Could you check a few things on this model? Use its own coordinates, in mm. A direction names the side the tool comes from. Coordinates: 2 decimals unless noted, no trailing zeros. Write each loop counter-clockwise with the first axis right and the second up, starting at its lowest first coordinate (ties: lowest second). Pieces come first, ordered by that corner, then holes.
Item 1: For P1, Ø5, axis at x = 0, z = 34, coming from the +Y side; P2, Ø2, axis at y = 0, z = -80, coming from the +X side; P3, Ø3, axis at x = 0, y = 0, coming from the +Z side; P4, Ø3, axis at x = 0, y = 0, coming from the -Z side, each with a flat end and sliding along its axis, tell me the tip position at first contact or that it passes through.
Item 2: Thinking about a two-plate mould opening in Y: for faces 1 (the flat face through (0, -5, -72)), 2 (the flat face through (2, 0.1, -32)), 3 (the cylindrical face through (-0.07, 0.07, -81.65)), 4 (the conical face through (0.3, 0.1, 93.7)), which applies, +Y half, -Y half, draft (parallel to the pull), parting line (faces both ways), or undercut?
Item 3: Which directions (+Z, -Z, +X, -X, +Y, -Y) give clear straight access to the entire face, cutting with the end or side of a thin tool? Please do faces 5 (the cylindrical face through (-1.216, 1.115, -100.17)), 6 (the flat face through (2, 0.1, 36)), 7 (the cylindrical face through (1.216, 1.115, 100.17)), 8 (the flat face through (2.3, -2, -33.9)), 9 (the flat face through (2, 0, -106)).
Item 4: I want a section at B-B on z = -34. Please give me the cut outline in (x, y).
Item 5: If I drill on probe 1 along Z at (x, y) = (0, 3.8); probe 2 along Z at (x, y) = (2.5, -4); probe 3 along X at (y, z) = (-1.4, 34), over which ranges is the centre line in solid material (lowest first)?
Item 6: I want a section at A-A on z = -4. Please give me the cut outline in (x, y), then the cut area to 3 significant figures.
from build123d import *

# Parameters (mm, degrees)
ESQUISSE1_W                                        = 10
ESQUISSE1_H                                        = 10
BOSS_EXTRU_1_DEPTH                                 = 106
TROU_TARAUD_M41_D                                  = 3.3
TROU_TARAUD_M41_DEPTH                              = 11.5
TROU_TARAUD_M41_TIP                                = 0.991420021
TROU_TARAUD_M42_D                                  = 3.3
TROU_TARAUD_M42_DEPTH                              = 11.5
TROU_TARAUD_M42_TIP                                = 0.991420021
CONG_1_R                                           = 2
CHAMBRAGE_POUR_VIS_T_TE_HEXAGONALE_M41_D           = 4.3
CHAMBRAGE_POUR_VIS_T_TE_HEXAGONALE_M41_CBORE_D     = 8
CHAMBRAGE_POUR_VIS_T_TE_HEXAGONALE_M41_CBORE_DEPTH = 4.9
ENL_V_MAT_EXTRU_1_REACH                            = 108.588
ESQUISSE8_W                                        = 10
ESQUISSE8_H                                        = 8
TROU_TARAUD_M44_D                                  = 3.3


with BuildPart() as part:
    # Esquisse1 → Boss.-Extru.1 (new, symmetric)
    with BuildSketch(Plane.XY):
        Rectangle(ESQUISSE1_W, ESQUISSE1_H)
    extrude(amount=BOSS_EXTRU_1_DEPTH, both=True)

    # Trou taraudé M41
    with Locations(Plane.XY.offset(106)):
        with Locations((0, 0)):
            Hole(TROU_TARAUD_M41_D / 2, depth=TROU_TARAUD_M41_DEPTH)
            with Locations((0, 0, -(TROU_TARAUD_M41_DEPTH + TROU_TARAUD_M41_TIP / 2))):  # 118° drill point
                Cone(0, TROU_TARAUD_M41_D / 2, TROU_TARAUD_M41_TIP, mode=Mode.SUBTRACT)

    # Trou taraudé M42
    with Locations(Plane(origin=(0, 0, -106), x_dir=(-1, 0, 0), z_dir=(0, 0, -1))):
        with Locations((0, 0)):
            Hole(TROU_TARAUD_M42_D / 2, depth=TROU_TARAUD_M42_DEPTH)
            with Locations((0, 0, -(TROU_TARAUD_M42_DEPTH + TROU_TARAUD_M42_TIP / 2))):  # 118° drill point
                Cone(0, TROU_TARAUD_M42_D / 2, TROU_TARAUD_M42_TIP, mode=Mode.SUBTRACT)

    # Congé1
    cong_1_edges = [part.edges().sort_by_distance(p)[0] for p in [
        (-5, 5, 0),
        (5, 5, 0),
        (5, -5, 0),
        (-5, -5, 0),
    ]]
    fillet(cong_1_edges, radius=CONG_1_R)

    # Chambrage pour vis à tête hexagonale M41 (through all)
    with Locations(Plane(origin=(0, 5, 0), x_dir=(1, 0, 0), z_dir=(0, 1, 0))):
        with Locations((0, 34), (0, -34)):
            CounterBoreHole(CHAMBRAGE_POUR_VIS_T_TE_HEXAGONALE_M41_D / 2, CHAMBRAGE_POUR_VIS_T_TE_HEXAGONALE_M41_CBORE_D / 2, CHAMBRAGE_POUR_VIS_T_TE_HEXAGONALE_M41_CBORE_DEPTH)

    # Esquisse8 → Enlèv. mat.-Extru.1 (cut, up to next)
    with BuildSketch(Plane(origin=(5, 0, 0), x_dir=(0, 0, -1), z_dir=(1, 0, 0)), mode=Mode.PRIVATE) as enl_v_mat_extru_1_sk1:
        with Locations((34, -6)):
            Rectangle(ESQUISSE8_W, ESQUISSE8_H)
    enl_v_mat_extru_1_tool1 = extrude(enl_v_mat_extru_1_sk1.sketch, amount=-ENL_V_MAT_EXTRU_1_REACH, mode=Mode.PRIVATE) & part.part
    # Esquisse8 → Enlèv. mat.-Extru.1 (cut, up to next)
    with BuildSketch(Plane(origin=(5, 0, 0), x_dir=(0, 0, -1), z_dir=(1, 0, 0)), mode=Mode.PRIVATE) as enl_v_mat_extru_1_sk2:
        with Locations((-34, -6)):
            Rectangle(ESQUISSE8_W, ESQUISSE8_H)
    enl_v_mat_extru_1_tool2 = extrude(enl_v_mat_extru_1_sk2.sketch, amount=-ENL_V_MAT_EXTRU_1_REACH, mode=Mode.PRIVATE) & part.part
    add(enl_v_mat_extru_1_tool1.solids().sort_by_distance((5, -6, -34))[0], mode=Mode.SUBTRACT)
    add(enl_v_mat_extru_1_tool2.solids().sort_by_distance((5, -6, 34))[0], mode=Mode.SUBTRACT)

    # Trou taraudé M44 (through all)
    with Locations(Plane(origin=(5, 0, 0), x_dir=(0, 0, -1), z_dir=(1, 0, 0))):
        with Locations((-80, 0), (80, 0)):
            Hole(TROU_TARAUD_M44_D / 2)


solid = part.part
Response values:
1. P1: stops at y = 0.1
1. P2: passes through
1. P3: stops at z = 94.41
1. P4: stops at z = -94.41
2. face 1: -Y half
2. face 2: +Y half
2. face 3: undercut
2. face 4: undercut
3. face 5: -Z
3. face 6: +Y
3. face 7: +Z
3. face 8: +X, -X, -Y
3. face 9: -Z, +X, -X, +Y, -Y
4. outline: (-5, -2) - (-2.15, -2) - (-2.15, 0.1) - (-4, 0.1) - (-4, 4.73) arc R2 ccw to (-5, 3) - close; (2.15, -2) - (5, -2) - (5, 3) arc R2 ccw to (4, 4.73) - (4, 0.1) - (2.15, 0.1) - close
5. probe 1: z = -106 to -38, -30 to 30, 38 to 106
5. probe 2: z = -106 to -39, -29 to 29, 39 to 106
5. probe 3: x = -5 to -2.15, 2.15 to 5
6. outline: (-5, -3) arc R2 ccw to (-3, -5) - (3, -5) arc R2 ccw to (5, -3) - (5, 3) arc R2 ccw to (3, 5) - (-3, 5) arc R2 ccw to (-5, 3) - close
6. area: 96.6 mm2
